CAD build for the part. Positions are in the model's coordinates, mm. Face numbers are marked on the shaded views. A direction names the side the tool comes from. Coordinates: 2 decimals unless noted, no trailing zeros. Loops run counter-clockwise (first coordinate to the right, second up) from the corner with the lowest first, then second, coordinate; pieces in that order, holes last. Notation, with made-up numbers: (-18.5, -8) -> (34.5, -8) arc R10 ccw to (34.5, 11) -> close; hole circle Ø11 at (74.25, 23). An arc over 180 degrees is marked (long way). Return JSON: item names as keys, results as strings. Group by question number.
(1) Saw through at C-C on x = -7. Write the cut outline in (y, z).
(2) Probe L1, parallel to X at y = 2, z = 28.5; L2, parallel to X at y = -11, z = 29.5; L3, parallel to X at y = -5, z = 30.5. List the from-to ranges inside material, lowest first.
(3) Flat gauge pins, fed straight in: pin 1 Ø10 at (y, z) = (5, 26.5) entering from -X; pin 2 Ø0.7 at (x, z) = (3.5, 18) entering from -Y; pin 3 Ø3 at (x, z) = (-17.5, 18.5) entering from -Y; pin 4 Ø8 at (x, y) = (-5, 8) entering from -Z. Where does each tip first touch, or does it go through?
(4) Tool access for the marked faces 4, 5 and 6: list every direction of +Z, -Z, +X, -X, +Y, -Y with a clear straight run to the whole face (end or side of a thin tool).
(5) Mould opens along X. For the marked faces 1, 2 and 3 say: pulls with the +X half, pulls with the -X half, needs draft (parallel to the pull), parting line crosses it, or undercut.
(6) Saw through at B-B on z = 17. Write the cut outline in (x, y).
(7) Saw through at D-D on y = -10. Write the cut outline in (x, z).
(8) Saw through at A-A on y = 7. Write the cut outline in (x, z).
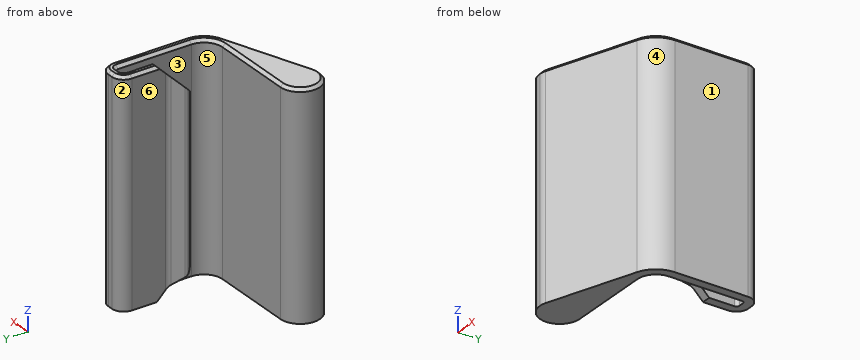
```python
from build123d import *

# Parameters (mm, degrees)
BOSS_EXTRUDE1_DEPTH = 60
CHAMFER2_SIZE       = 0.8
CUT_EXTRUDE1_DEPTH  = 73.196490998
FILLET2_R           = 0.8


with BuildPart() as part:
    # Sketch1 → Boss-Extrude1 (new body)
    with BuildSketch(Plane.XY):
        with BuildLine():
            Line((2.4, 0), (2.4, 9.2))
            ThreePointArc((2.4, 9.2), (2.634314575, 9.765685425), (3.2, 10))
            Line((3.2, 10), (4.6, 10))
            ThreePointArc((4.6, 10), (5.165685425, 9.765685425), (5.4, 9.2))
            Line((5.4, 9.2), (5.4, -10.8))
            ThreePointArc((5.4, -10.8), (3.935533906, -14.335533906), (0.4, -15.8))
            Line((0.4, -15.8), (-22.271467176, -15.8))
            ThreePointArc((-22.271467176, -15.8), (-27.674350112, -21.202882937), (-22.271467176, -26.605765873))
            ThreePointArc((-22.271467176, -26.605765873), (-21.403226287, -26.529804638), (-20.561366459, -26.304228977))
            Line((-20.561366459, -26.304228977), (2.930949061, -17.753725394))
            ThreePointArc((2.930949061, -17.753725394), (6.461725128, -15.044465629), (7.8, -10.8))
            Line((7.8, -10.8), (7.8, 9.2))
            ThreePointArc((7.8, 9.2), (6.8627417, 11.4627417), (4.6, 12.4))
            Line((4.6, 12.4), (3.2, 12.4))
            ThreePointArc((3.2, 12.4), (0.9372583, 11.4627417), (0, 9.2))
            Line((0, 9.2), (0, 0))
            ThreePointArc((0, 0), (-0.121792748, -0.612293492), (-0.46862915, -1.13137085))
            Line((-0.46862915, -1.13137085), (-3.297056275, -3.959797975))
            Line((-3.297056275, -3.959797975), (-1.6, -5.656854249))
            Line((-1.6, -5.656854249), (1.228427125, -2.828427125))
            ThreePointArc((1.228427125, -2.828427125), (2.09551813, -1.530733729), (2.4, 0))
        make_face()
    extrude(amount=BOSS_EXTRUDE1_DEPTH)

    # Chamfer2
    chamfer2_edges = [part.edges().sort_by_distance(p)[0] for p in [
        (-0.185786438, -4.242640687, 60),
        (2.09551813, -1.530733729, 60),
        (2.4, 4.6, 60),
        (2.634314575, 9.765685425, 60),
        (3.9, 10, 60),
        (5.165685425, 9.765685425, 60),
        (5.4, -0.8, 60),
        (3.935533906, -14.335533906, 60),
        (-10.935733588, -15.8, 60),
        (-0.121792748, -0.612293492, 60),
        (-27.674350112, -21.202882937, 60),
        (-21.403226287, -26.529804638, 60),
        (-8.815208699, -22.028977185, 60),
        (6.461725128, -15.044465629, 60),
        (7.8, -0.8, 60),
        (6.8627417, 11.4627417, 60),
        (3.9, 12.4, 60),
        (0.9372583, 11.4627417, 60),
        (0, 4.6, 60),
        (-1.882842712, -2.545584412, 60),
    ]]
    chamfer(chamfer2_edges, length=CHAMFER2_SIZE)

    # Sketch2 → Cut-Extrude1 (cut, through all)
    with BuildSketch(Plane(origin=(2.4, 0, 0), x_dir=(0, 0, -1), z_dir=(1, 0, 0))):
        Polygon((-60, 2.343145751), (-52, -5.656854249), (-60, -5.656854249), align=None)
        Polygon((0, 2.343145751), (-8, -5.656854249), (0, -5.656854249), align=None)
    extrude(amount=-CUT_EXTRUDE1_DEPTH, mode=Mode.SUBTRACT)

    # Fillet2
    fillet2_edges = [part.edges().sort_by_distance(p)[0] for p in [
        (-1.6, -5.656854249, 30),
        (-3.297056275, -3.959797975, 30),
    ]]
    fillet(fillet2_edges, radius=FILLET2_R)


solid = part.part
```
Geometry results:
{
 "1": {"outline": "(-21.37, 0) -> (-15.8, 0) -> (-15.8, 59.2) -> (-16.6, 60) -> (-20.52, 60) -> (-21.37, 59.2) -> close"},
 "2": {"L1": "0 to 2.4, 5.4 to 7.8", "L2": "5.4 to 7.8", "L3": "-2.26 to -0.94, 5.4 to 7.8"},
 "3": {"pin 1": "x = 0", "pin 2": "y = -17.67", "pin 3": "y = -25.74", "pin 4": "through"},
 "4": {"face 4": "+Z, -Z, +X, -Y", "face 5": "+Z, -Z, -X", "face 6": "+Z, -Z, -X, +Y"},
 "5": {"face 1": "pulls with the +X half", "face 2": "pulls with the -X half", "face 3": "undercut"},
 "6": {"outline": "(-22.27, -26.61) arc R5 ccw to (-20.56, -26.3) -> (2.93, -17.75) arc R7.4 ccw to (7.8, -10.8) -> (7.8, 9.2) arc R3.2 ccw to (4.6, 12.4) -> (3.2, 12.4) arc R3.2 ccw to (0, 9.2) -> (0, 0) arc R1.6 cw to (-0.47, -1.13) -> (-2.73, -3.39) arc R0.8 ccw to (-2.73, -4.53) -> (-2.17, -5.09) arc R0.8 ccw to (-1.03, -5.09) -> (1.23, -2.83) arc R4 ccw to (2.4, 0) -> (2.4, 9.2) arc R0.8 cw to (3.2, 10) -> (4.6, 10) arc R0.8 cw to (5.4, 9.2) -> (5.4, -10.8) arc R5 cw to (0.4, -15.8) -> (-22.27, -15.8) arc R5.4 ccw to start"},
 "7": {"outline": "(5.4, 0) -> (7.8, 0) -> (7.8, 59.2) -> (7, 60) -> (6.2, 60) -> (5.4, 59.2) -> close"},
 "8": {"outline": "(0, 0) -> (2.4, 0) -> (2.4, 59.2) -> (1.6, 60) -> (0.8, 60) -> (0, 59.2) -> close; (5.4, 0) -> (7.8, 0) -> (7.8, 59.2) -> (7, 60) -> (6.2, 60) -> (5.4, 59.2) -> close"}
}
